Read the model definition and answer for the solid it produces. Units are mm, in the model's axes. A direction names the side the tool comes from. Coordinates: 2 decimals unless noted, no trailing zeros. Write each loop counter-clockwise with the first axis right and the second up, starting at its lowest first coordinate (ties: lowest second). Pieces come first, ordered by that corner, then holes.
(1) Section C-C on x = 1.5 is taken. Write down the section's boundary in (y, z), then the cut area to 3 significant figures.
(2) Section B-B on y = 2 is taken. Write down the section's boundary in (x, z), then the cut area to 3 significant figures.
(3) Find the intervals of material crossed by probe 1 along Y at (x, z) = (1, 26); probe 2 along X at (y, z) = (7.25, 23.5); probe 3 along X at (y, z) = (3, 11.5), in increasing order.
(4) Section A-A on z = 15.5 is taken. Write down the section's boundary in (x, y).
(5) Which of the six approach directions +Z, -Z, +X, -X, +Y, -Y give full straight-line access (tool end or side, diameter ignored) to faces 1 (the flat face through (0, -8.379, 15)), 2 (the flat face through (0, 0, 30)), 3 (the flat face through (0, 8.379, 15))?
(6) The mould has two halves that part along Y. Classify faces 4 (the flat face through (0, 0, 0)), 5 (the cylindrical face through (4.533, 7.775, 14.79)), 6 (the cylindrical face through (-4.533, -7.775, 14.79)), 7 (the cylindrical face through (9, 0, 15)): +Y half, -Y half, draft (parallel to the pull), parting line (faces both ways), or undercut.
(7) Given pin 1 (5 mm diameter, centred on x = -5.5, z = 4, fed in from +Y); pin 2 (5 mm diameter, centred on y = 5, z = 18.5, fed in from -X); pin 3 (1 mm diameter, centred on y = -4, z = 12.5, fed in from +X), each flat-ended and moving along its own axis, determine where each tip first touches the part or whether it passes through.
from build123d import *

# Parameters (mm, degrees)
F1_DEPTH = 30


with BuildPart() as f1:
    # F0 (on Top) → F1 (new body)
    with BuildSketch(Plane.XY):
        with BuildLine():
            Line((2, -8.379183), (2, -8.774964))
            ThreePointArc((2, -8.774964), (4.5, -7.794229), (6.599342, -6.119533))
            Line((6.599342, -6.119533), (6.256585, -5.921642))
            Line((6.256585, -5.921642), (8.256585, -2.457541))
            Line((8.256585, -2.457541), (8.599342, -2.655431))
            ThreePointArc((8.599342, -2.655431), (9, 0), (8.599342, 2.655431))
            Line((8.599342, 2.655431), (8.256585, 2.457541))
            Line((8.256585, 2.457541), (6.256585, 5.921642))
            Line((6.256585, 5.921642), (6.599342, 6.119533))
            ThreePointArc((6.599342, 6.119533), (4.5, 7.794229), (2, 8.774964))
            Line((2, 8.774964), (2, 8.379183))
            Line((2, 8.379183), (-2, 8.379183))
            Line((-2, 8.379183), (-2, 8.774964))
            ThreePointArc((-2, 8.774964), (-4.5, 7.794229), (-6.599342, 6.119533))
            Line((-6.599342, 6.119533), (-6.256585, 5.921642))
            Line((-6.256585, 5.921642), (-8.256585, 2.457541))
            Line((-8.256585, 2.457541), (-8.599342, 2.655431))
            ThreePointArc((-8.599342, 2.655431), (-9, 0), (-8.599342, -2.655431))
            Line((-8.599342, -2.655431), (-8.256585, -2.457541))
            Line((-8.256585, -2.457541), (-6.256585, -5.921642))
            Line((-6.256585, -5.921642), (-6.599342, -6.119533))
            ThreePointArc((-6.599342, -6.119533), (-4.5, -7.794229), (-2, -8.774964))
            Line((-2, -8.774964), (-2, -8.379183))
            Line((-2, -8.379183), (2, -8.379183))
        make_face()
    extrude(amount=F1_DEPTH)


solid = f1.part
Response:
1. outline: (-8.38, 0) - (8.38, 0) - (8.38, 30) - (-8.38, 30) - close
1. area: 503 mm2
2. outline: (-8.77, 0) - (8.77, 0) - (8.77, 30) - (-8.77, 30) - close
2. area: 526 mm2
3. probe 1: y = -8.38 to 8.38
3. probe 2: x = -5.33 to 5.33
3. probe 3: x = -7.94 to 7.94
4. outline: (-8.6, -2.66) - (-8.26, -2.46) - (-6.26, -5.92) - (-6.6, -6.12) arc R9 ccw to (-2, -8.77) - (-2, -8.38) - (2, -8.38) - (2, -8.77) arc R9 ccw to (6.6, -6.12) - (6.26, -5.92) - (8.26, -2.46) - (8.6, -2.66) arc R9 ccw to (8.6, 2.66) - (8.26, 2.46) - (6.26, 5.92) - (6.6, 6.12) arc R9 ccw to (2, 8.77) - (2, 8.38) - (-2, 8.38) - (-2, 8.77) arc R9 ccw to (-6.6, 6.12) - (-6.26, 5.92) - (-8.26, 2.46) - (-8.6, 2.66) arc R9 ccw to start
5. face 1: +Z, -Z, -Y
5. face 2: +Z, +X, -X, +Y, -Y
5. face 3: +Z, -Z, +Y
6. face 4: draft
6. face 5: +Y half
6. face 6: -Y half
6. face 7: parting line
7. pin 1: stops at y = 8.49
7. pin 2: stops at x = -8.65
7. pin 3: stops at x = 7.65
